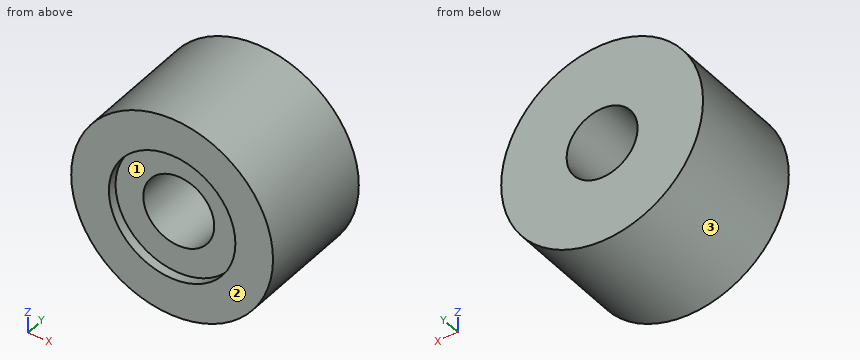
from build123d import *

# Parameters (mm, degrees)
F0_R     = 4.45
F0_R_2   = 2.79
F1_DEPTH = 5.42
F0_R_3   = 1.565
F2_DEPTH = 5
F3_DEPTH = 5.42


with BuildPart() as f1:
    # F0 (on Front) → F1 (new body)
    with BuildSketch(Plane.XZ):
        with Locations((-44.581614, 35.172123)):
            Circle(F0_R)
        with Locations((-44.581614, 35.172123)):
            Circle(F0_R_2, mode=Mode.SUBTRACT)
    extrude(amount=F1_DEPTH)

    # F0 (on Front) → F2 (join)
    with BuildSketch(Plane.XZ):
        with Locations((-44.581614, 35.172123)):
            Circle(F0_R_2)
        with Locations((-44.581614, 35.172123)):
            Circle(F0_R_3, mode=Mode.SUBTRACT)
    extrude(amount=F2_DEPTH)

    # F0 (on Front) → F3 (cut)
    with BuildSketch(Plane.XZ):
        with Locations((-44.581614, 35.172123)):
            Circle(F0_R_3)
    extrude(amount=-F3_DEPTH, mode=Mode.SUBTRACT)


solid = f1.part
The model under review builds one solid part; all positions refer to its coordinate system, in mm. Face numbers are marked on the shaded views. Give positions to 0.01 mm unless a question says otherwise; leave off trailing zeros. Write each loop counter-clockwise with the first axis right and the second up, starting at its lowest first coordinate (ties: lowest second). Pieces come first, ordered by that corner, then holes.
1. Draft analysis for pull direction X (two halves, no side actions). For the marked faces 1, 2 and 3, state which applies: +X half, -X half, draft (parallel to the pull), parting line (faces both ways), or undercut.
2. For P1, Ø1, axis at x = -46, y = -2.5, coming from the -Z side; P2, Ø1.7, axis at x = -46, z = 36, coming from the -Y side; P3, Ø2, axis at x = -47, y = -4, coming from the -Z side, all flat-tipped, find the tip position at first contact; note any pin that passes through.
3. Add section B-B, the plane z = 37.5. Write out the cut boundary in (x, y).
4. Add section A-A, the plane x = -45.75. Write out the cut boundary in (y, z).
5. Wall thickness on L1, parallel to Y at x = -42.75, z = 35.5; L2, parallel to Z at x = -46, y = -4.55; L3, parallel to Z at x = -44, y = -0.75: over which ranges is each line inside the solid? List them lowest first.
6. Add section D-D, the plane x = -44.75. Write out the cut boundary in (y, z).
7. Add section C-C, the plane x = -46.75. Write out the cut boundary in (y, z).
Worked answers:
1. face 1: undercut
1. face 2: draft
1. face 3: parting line
2. P1: stops at z = 30.82
2. P2: stops at y = -5
2. P3: stops at z = 30.95
3. outline: (-48.37, -5.42) - (-46.12, -5.42) - (-46.12, -5) - (-43.04, -5) - (-43.04, -5.42) - (-40.79, -5.42) - (-40.79, 0) - (-48.37, 0) - close
4. outline: (-5.42, 30.88) - (0, 30.88) - (0, 34.13) - (-5, 34.13) - (-5, 32.64) - (-5.42, 32.64) - close; (-5.42, 37.71) - (-5, 37.71) - (-5, 36.21) - (0, 36.21) - (0, 39.47) - (-5.42, 39.47) - close
5. L1: y = -5 to 0
5. L2: z = 30.95 to 34.51, 35.83 to 39.39
5. L3: z = 30.76 to 33.72, 36.63 to 39.58
6. outline: (-5.42, 30.73) - (0, 30.73) - (0, 33.62) - (-5, 33.62) - (-5, 32.39) - (-5.42, 32.39) - close; (-5.42, 37.96) - (-5, 37.96) - (-5, 36.73) - (0, 36.73) - (0, 39.62) - (-5.42, 39.62) - close
7. outline: (-5.42, 31.29) - (0, 31.29) - (0, 39.06) - (-5.42, 39.06) - (-5.42, 36.93) - (-5, 36.93) - (-5, 33.42) - (-5.42, 33.42) - close
